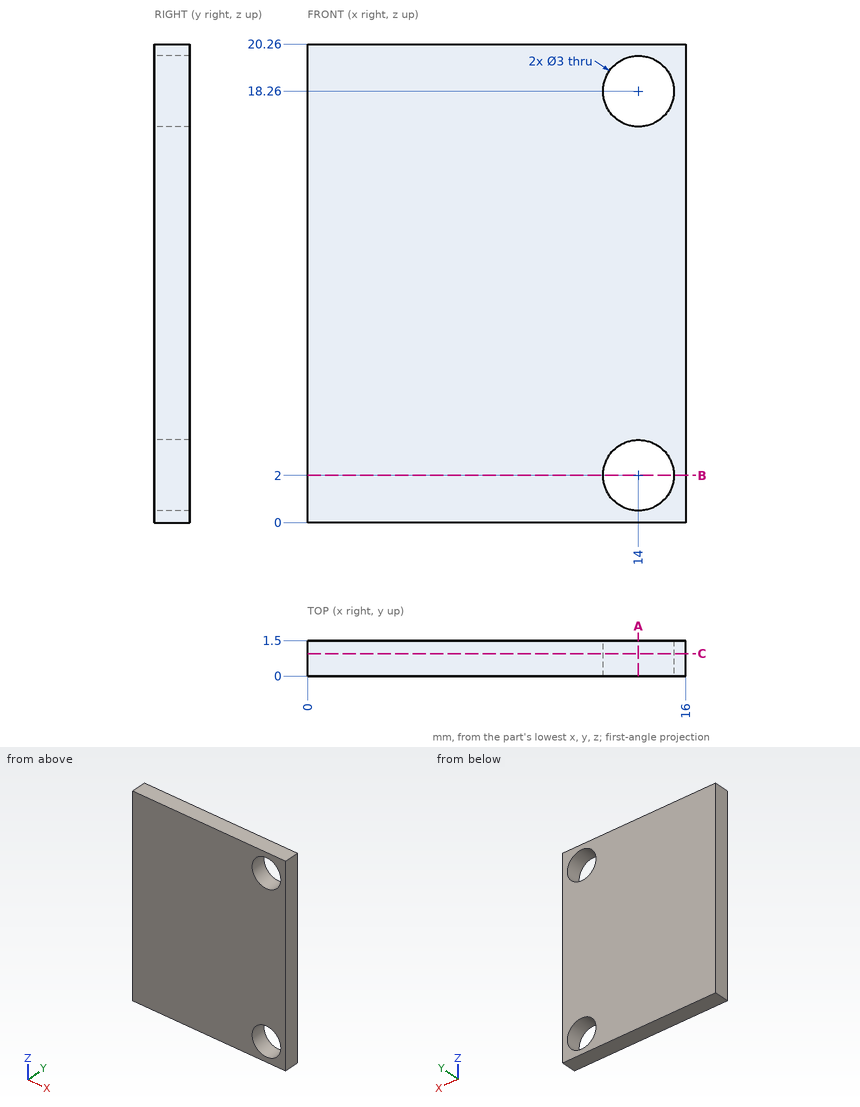
Geometry: see drawing. Coordinates: mm, zero at the bounding-box minimum. Round coordinates to 2 decimals unless told otherwise and drop trailing zeros. Order: outer loops, then holes, each group sorted by start corner. A loop starts at its lowest first (then second) coordinate and runs counter-clockwise, first axis right, second up. Notation, with made-up numbers: (44.25, 44.5) - (84.25, 44.5) arc R9 cw to (84.25, 52.5) - close; hole circle Ø4 at (50, 67). An arc over 180 degrees is marked (long way). One line per question, with ' | ' between items. Start each with the question number.
1) Ray query, probe 1 along Z at (x, y) = (14, 0.9); probe 2 along Z at (x, y) = (13.5, 1.3); probe 3 along X at (y, z) = (0.6, 2.25). Return the intervals inside material, ascending.
2) Cut plane A-A, the plane x = 14. Return the cut outline in (y, z), then the cut area to 3 significant figures.
3) Cut plane C-C, the plane y = 0.95. Return the cut outline in (x, z).
4) Cut plane B-B, the plane z = 2. Return the cut outline in (x, y).
Worked out:
1) probe 1: z = 0 to 0.5, 3.5 to 16.76, 19.76 to 20.26 | probe 2: z = 0 to 0.59, 3.41 to 16.85, 19.67 to 20.26 | probe 3: x = 0 to 12.52, 15.48 to 16
2) outline: (0, 0) - (1.5, 0) - (1.5, 0.5) - (0, 0.5) - close; (0, 3.5) - (1.5, 3.5) - (1.5, 16.76) - (0, 16.76) - close; (0, 19.76) - (1.5, 19.76) - (1.5, 20.26) - (0, 20.26) - close | area: 21.4 mm^2
3) outline: (0, 0) - (16, 0) - (16, 20.26) - (0, 20.26) - close; hole circle Ø3 at (14, 2); hole circle Ø3 at (14, 18.26)
4) outline: (0, 0) - (12.5, 0) - (12.5, 1.5) - (0, 1.5) - close; (15.5, 0) - (16, 0) - (16, 1.5) - (15.5, 1.5) - close
